Geometry check sheet. Reference: the model listing, model coordinates, mm. Round coordinates to 2 decimals unless told otherwise and drop trailing zeros. Order: outer loops, then holes, each group sorted by start corner. A loop starts at its lowest first (then second) coordinate and runs counter-clockwise, first axis right, second up. Notation, with made-up numbers: (74, 22) -> (98, 22) arc R26 cw to (98, 46) -> close; hole circle Ø6 at (59, 56.5). An arc over 180 degrees is marked (long way). Use a Markdown table: item, result. Add a question column.
Item 1: Sectioned sample at B-B, the plane x = 15. Record the cut outline in (y, z), and give its area (4 significant figures).
Item 2: Gauge pin test, flat ends, axial feed: pin 1 Ø1.9 at (x, y) = (15, 0) entering from +Z; pin 2 Ø4 at (x, y) = (-15, 4) entering from -Z. Record the tip position at first contact, or that the pin passes through.
Item 3: Mould release check, pull along Y, two halves, no side actions. Record for faces 1 (the cylindrical face through (6.875, -0.715, 0.74)), 2 (the flat face through (20, 0, 1)), 3 (the flat face through (0, -5, 1)): pulls with the +Y half, pulls with the -Y half, needs draft (parallel to the pull), parting line crosses it, or undercut.
Item 4: Material ranges on probe 1 along X at (y, z) = (0, 1.15); probe 2 along Y at (x, z) = (-15, 0.65); probe 3 along X at (y, z) = (-1.25, 0.95), recorded low to high. Write a range as [from, to].
Item 5: Sectioned sample at A-A, the plane y = 0. Record the cut outline in (x, z).
Item 6: Sectioned sample at C-C, the plane z = 0.85. Record the cut outline in (x, y), and give its area (3 significant figures).
Item 7: Sectioned sample at D-D, the plane x = 5.5. Record the cut outline in (y, z), and give its area (4 significant figures).
Autodesk Inventor part; units mm, degrees
ref_plane "YZ Plane" through (0, 0, 0) normal (1, 0, 0) x (0, 1, 0)
ref_plane "XZ Plane" through (0, 0, 0) normal (0, 1, 0) x (-1, 0, 0)
ref_plane "XY Plane" through (0, 0, 0) normal (0, 0, 1) x (1, 0, 0)
sketch "スケッチ1" plane through (0, 0, 0) normal (0, 0, 1) x (1, 0, 0)
  line L0 (-20, 5) -> (20, 5)
  line L1 (20, 5) -> (20, -5)
  line L2 (20, -5) -> (-20, -5)
  line L3 (-20, -5) -> (-20, 5)
  line L4 (-20, 5) -> (20, -5) construction
  line L5 (20, 5) -> (-20, -5) construction
  point P0 (0, 0)
  dimension "d0" = 40
  dimension "d1" = 10
extrude "押し出し1" add sketch "スケッチ1" along normal blind 1.5
sketch "スケッチ2" plane through (0, 0, 1.5) normal (0, 0, 1) x (1, 0, 0)
  point P0 (0, 0)
  point P1 (-5.5, 0)
  point P2 (5.5, 0)
  dimension "d4" = 0
  dimension "d5" = 11
  dimension "d6" = 5.5
hole "穴1" at (-5.5, 0, 1.5) at (5.5, 0, 1.5) direction (0, 0, -1) diameter 3.1 end through all
sketch "スケッチ3" plane through (0, 0, 1.5) normal (0, 0, 1) x (1, 0, 0)
  line L0 (20, -5) -> (20, 5)
  line L1 (-20, 5) -> (-20, -5)
  point P0 (0, 0)
  point P1 (-15, 0)
  point P2 (15, 0)
  dimension "d14" = 5
  dimension "d15" = 5
hole "穴2" at (-15, 0, 1.5) at (15, 0, 1.5) direction (0, 0, -1) diameter 2.1 end through all
properties material "アルミニウム 5052 H32"
Found:
| question | item | result |
|---|---|---|
| 1 | outline | (-5, 0) -> (-1.05, 0) -> (-1.05, 1.5) -> (-5, 1.5) -> close; (1.05, 0) -> (5, 0) -> (5, 1.5) -> (1.05, 1.5) -> close |
| 1 | area | 11.85 mm2 |
| 2 | pin 1 | passes through |
| 2 | pin 2 | stops at z = 0 |
| 3 | face 1 | undercut |
| 3 | face 2 | needs draft |
| 3 | face 3 | pulls with the -Y half |
| 4 | probe 1 | x = [-20, -16.05], [-13.95, -7.05], [-3.95, 3.95], [7.05, 13.95], [16.05, 20] |
| 4 | probe 2 | y = [-5, -1.05], [1.05, 5] |
| 4 | probe 3 | x = [-20, -6.42], [-4.58, 4.58], [6.42, 20] |
| 5 | outline | (-20, 0) -> (-16.05, 0) -> (-16.05, 1.5) -> (-20, 1.5) -> close; (-13.95, 0) -> (-7.05, 0) -> (-7.05, 1.5) -> (-13.95, 1.5) -> close; (-3.95, 0) -> (3.95, 0) -> (3.95, 1.5) -> (-3.95, 1.5) -> close; (7.05, 0) -> (13.95, 0) -> (13.95, 1.5) -> (7.05, 1.5) -> close; (16.05, 0) -> (20, 0) -> (20, 1.5) -> (16.05, 1.5) -> close |
| 6 | outline | (-20, -5) -> (20, -5) -> (20, 5) -> (-20, 5) -> close; hole circle Ø2.1 at (-15, 0); hole circle Ø3.1 at (-5.5, 0); hole circle Ø3.1 at (5.5, 0); hole circle Ø2.1 at (15, 0) |
| 6 | area | 378 mm2 |
| 7 | outline | (-5, 0) -> (-1.55, 0) -> (-1.55, 1.5) -> (-5, 1.5) -> close; (1.55, 0) -> (5, 0) -> (5, 1.5) -> (1.55, 1.5) -> close |
| 7 | area | 10.35 mm2 |
